```python
from build123d import *

# Parameters (mm, degrees)
SKETCH_1_W               = 34
SKETCH_1_H               = 28
EXTRUDE_1_DEPTH          = 6
CUT_EXTRUDE_1_DEPTH      = 42.949279402
CUT_EXTRUDE_1_DEPTH_BACK = 42.949279402
CUT_EXTRUDE_3_REACH      = 33.664
SKETCH_5_R               = 4
SKETCH_9_W               = 5
SKETCH_9_H               = 12
EXTRUDE_4_DEPTH          = 20
CUT_EXTRUDE_4_REACH      = 40.227
SKETCH_10_R              = 4


with BuildPart() as part:
    # 草图1 → 凸台-拉伸1 (new body)
    with BuildSketch(Plane(origin=(0, 0, 0), x_dir=(1, 0, 0), z_dir=(0, 1, 0))):
        with Locations((2.971223022, 9.827338129)):
            Rectangle(SKETCH_1_W, SKETCH_1_H)
    extrude(amount=EXTRUDE_1_DEPTH)

    # 草图2 → 切除-拉伸1 (cut, two sides: drawn at the far end of the back side and taken through both)
    with BuildSketch(Plane(origin=(19.971223022, 0, 0), x_dir=(0, 0, -1), z_dir=(1, 0, 0)).offset(-CUT_EXTRUDE_1_DEPTH_BACK)):
        Polygon((90.395880624, 2), (23.827338129, 2), (5.827338129, 2), (5.827338129, 0), (5.827338129, -66.568542495), (89.676932139, -169.983865267), (174.245474634, -101.415322772), align=None)
    extrude(amount=CUT_EXTRUDE_1_DEPTH + CUT_EXTRUDE_1_DEPTH_BACK, mode=Mode.SUBTRACT)

    # 草图5 → 切除-拉伸3 (cut, up to next)
    with BuildSketch(Plane.XZ, mode=Mode.PRIVATE) as cut_extrude_3_sk1:
        with Locations(Location((-9.028776978, -0.827338129, 0), (0, 0, 270))):
            Circle(SKETCH_5_R)
    cut_extrude_3_tool1 = extrude(cut_extrude_3_sk1.sketch, amount=-CUT_EXTRUDE_3_REACH, mode=Mode.PRIVATE) & part.part
    # 草图5 → 切除-拉伸3 (cut, up to next)
    with BuildSketch(Plane.XZ, mode=Mode.PRIVATE) as cut_extrude_3_sk2:
        with Locations(Location((14.971223022, -0.827338129, 0), (0, 0, 270))):
            Circle(SKETCH_5_R)
    cut_extrude_3_tool2 = extrude(cut_extrude_3_sk2.sketch, amount=-CUT_EXTRUDE_3_REACH, mode=Mode.PRIVATE) & part.part
    add(cut_extrude_3_tool1.solids().sort_by_distance((-9.028777, 0, -0.827338))[0], mode=Mode.SUBTRACT)
    add(cut_extrude_3_tool2.solids().sort_by_distance((14.971223, 0, -0.827338))[0], mode=Mode.SUBTRACT)

    # 草图9 → 凸台-拉伸4 (add)
    with BuildSketch(Plane.XY.offset(4.172661871)):
        with Locations((-11.528776978, 0)):
            Rectangle(SKETCH_9_W, SKETCH_9_H)
    extrude(amount=EXTRUDE_4_DEPTH)

    # 草图10 → 切除-拉伸4 (cut, up to next)
    with BuildSketch(Plane(origin=(-9.028776978, 0, 0), x_dir=(0, 0, -1), z_dir=(1, 0, 0)), mode=Mode.PRIVATE) as cut_extrude_4_sk1:
        with Locations(Location((-17.172661871, 0, 0), (0, 0, 90))):
            Circle(SKETCH_10_R)
    cut_extrude_4_tool1 = extrude(cut_extrude_4_sk1.sketch, amount=-CUT_EXTRUDE_4_REACH, mode=Mode.PRIVATE) & part.part
    add(cut_extrude_4_tool1.solids().sort_by_distance((-9.028777, 0, 17.172662))[0], mode=Mode.SUBTRACT)


solid = part.part
```
For this review, take the finished solid that the model builds, in its own axes (mm). A direction names the side the tool comes from. Coordinates: 2 decimals unless noted, no trailing zeros. Write each loop counter-clockwise with the first axis right and the second up, starting at its lowest first coordinate (ties: lowest second). Pieces come first, ordered by that corner, then holes.
(1) Add section B-B on x = -11. Give the boundary of the cut face in (y, z), then the cut area to 3 significant figures.
(2) The part is to be moulded in two halves that separate along Z. For faces 1 (the face through (3, 1, -5.827)), 2 (the face through (19.971, 4, -10)), 3 (the face through (-11.49, -0.87, 13.27)), say which applies: +Z half, -Z half, draft (parallel to the pull), parting line (faces both ways), or undercut.
(3) For pin 1 Ø1 at (x, y) = (9.5, 0.5) entering from -Z; pin 2 Ø3 at (x, z) = (11, 0.5) entering from -Y; pin 3 Ø5 at (x, y) = (7, 1.5) entering from +Z, all flat-tipped, find the tip position at first contact; note any pin that passes through.
(4) Tool access review of faces 4 (the face through (-9.029, 0, 12)), 5 (the face through (3, 2, -15)), 6 (the face through (-12, -6, 14)): name each direction out of +Z, -Z, +X, -X, +Y, -Y from which nothing blocks a thin tool from reaching the whole face with its end or side.
(5) Add section C-C on z = -0.5. Give the boundary of the cut face in (x, y).
(6) Wall thickness on probe 1 along Z at (x, y) = (-9.5, 3); probe 2 along X at (y, z) = (1, -3); probe 3 along X at (y, z) = (0, 8): over which ranges is each line inside the solid? List them lowest first.
(7) Add section D-D on x = -7.5. Give the boundary of the cut face in (y, z).
(8) Add section A-A on y = 3. Give the boundary of the cut face in (x, z), then the cut area to 3 significant figures.
Answer sheet:
1. outline: (-6, 4.17) - (0, 4.17) - (0, 2.65) - (6, 2.65) - (6, 24.17) - (-6, 24.17) - close; (0, -5.83) - (2, -5.83) - (2, -23.83) - (6, -23.83) - (6, -4.31) - (0, -4.31) - close; hole circle Ø8 at (0, 17.17)
1. area: 280 mm2
2. face 1: -Z half
2. face 2: draft
2. face 3: undercut
3. pin 1: stops at z = -5.83
3. pin 2: stops at y = 0
3. pin 3: stops at z = 4.17
4. face 4: +Z, +X, +Y, -Y
4. face 5: -Z, +X, -X, -Y
4. face 6: +Z, -Z, +X, -X, -Y
5. outline: (-14.03, 0) - (-13.02, 0) - (-13.02, 6) - (-14.03, 6) - close; (-5.04, 0) - (10.98, 0) - (10.98, 6) - (-5.04, 6) - close; (18.96, 0) - (19.97, 0) - (19.97, 6) - (18.96, 6) - close
6. probe 1: z = -23.83 to -4.8, 3.14 to 14.53, 19.82 to 24.17
6. probe 2: x = -14.03 to -12.39, -5.67 to 11.61, 18.33 to 19.97
6. probe 3: x = -14.03 to -9.03
7. outline: (0, -5.83) - (2, -5.83) - (2, -23.83) - (6, -23.83) - (6, -4.52) - (0, -4.52) - close; (0, 2.87) - (6, 2.87) - (6, 4.17) - (0, 4.17) - close
8. outline: (-14.03, -23.83) - (19.97, -23.83) - (19.97, 4.17) - (-9.03, 4.17) - (-9.03, 14.53) - (-14.03, 14.53) - close; (-14.03, 19.82) - (-9.03, 19.82) - (-9.03, 24.17) - (-14.03, 24.17) - close; hole circle Ø8 at (-9.03, -0.83); hole circle Ø8 at (14.97, -0.83)
8. area: 925 mm2
